Input: part model. Units: mm. Frame: model coordinates. A direction names the side the tool comes from. Give positions to 0.01 mm unless a question says otherwise; leave off trailing zeros. Write each loop counter-clockwise with the first axis right and the second up, starting at its lowest first coordinate (ties: lowest second). Pieces come first, ordered by that corner, then holes. Notation, with made-up numbers: (4.5, 44) - (39.5, 44) arc R19 cw to (39.5, 77) - close; hole circle Ø11 at (31, -15.5). An arc over 180 degrees is marked (long way). Use a Markdown table: item, result. Add a question column.
1. Section query D-D, the plane y = 29.5. Return loops of the section in (x, z).
2. Mould query, pull axis Y, two halves, no side actions, for faces 1 (the flat face through (-36, 20, 47)), 2 (the flat face through (-13, -22, 5)), 3 (the conical face through (-32.96, 35.88, 89.19)). Classes: released by +Y, released by -Y, zero draft, split by the parting line, or undercut.
3. Set-up query: faces 4 (the cylindrical face through (-7.262, -32.703, 45.56)), 5 (the cylindrical face through (2.769, -34.504, 9.677)), 6 (the flat face through (16, 30, 85)). Return all of +Z, -Z, +X, -X, +Y, -Y with unobstructed straight access to the full face (end or side cutting, diameter ignored); none if empty.
4. Pin query (flat end, axial travel): pin 1 (3 mm diameter, centred on x = 4, z = 16, fed in from -Y); pin 2 (2.5 mm diameter, centred on x = -31, z = 90, fed in from +Y); pin 3 (12 mm diameter, centred on x = 23, z = 40.5, fed in from -Y); pin 4 (5 mm diameter, centred on x = -3.5, z = 12.5, fed in from -Y). Return the tip coordinate at first contact, or that it passes through.
5. Section query A-A, the plane z = 90. Return loops of the section in (x, y), plus the area to 4 significant figures.
6. Material intervals for probe 1 along X at (y, z) = (37.1, 90); probe 2 along Y at (x, z) = (0, 30); probe 3 along Z at (x, y) = (-31, 37.4), sorted ascending.
7. Section query C-C, the plane y = 21. Return loops of the section in (x, z).
8. Section query B-B, the plane x = -31. Return loops of the section in (y, z), plus the area to 3 significant figures.
```python
from build123d import *
from build123d import SkipClean  # not in build123d's __all__

# Parameters (mm, degrees)
F1_DEPTH        = 95
F2_W            = 72
F2_H            = 80
F3_DEPTH        = 10
F4_R            = 33.5
F5_DEPTH        = 80
F7_D            = 4
F7_CSINK_D      = 9
F7_CSINK_ANGLE  = 90
F7_COPIES_COUNT = 2
F7_COPIES_PITCH = 81.154174
F8_R            = 25
F9_DEPTH        = 5.001
F11_R           = 6
F12_DEPTH       = 73.5


# Not quite as in the source:
# - a feature of the source that left no trace in its solid (it failed there, or was rolled back) is left out
# - a pattern or mirror of a feature is missing from the dataset's text; its kind, count and spacing are read off the source's solid


with BuildPart() as f1:
    # F0 (on Top) → F1 (new body)
    with BuildSketch(Plane.XY):
        with BuildLine():
            Line((36, 38.5), (-36, 38.5))
            Line((-36, 38.5), (-36, 0))
            ThreePointArc((-36, 0), (0, -36), (36, 0))
            Line((36, 0), (36, 38.5))
        make_face()
    extrude(amount=F1_DEPTH)

    # F2 (on face) → F3 (cut)
    with BuildSketch(Plane.XY.offset(95)):
        with Locations((0, -6.5)):
            Rectangle(F2_W, F2_H)
    extrude(amount=-F3_DEPTH, mode=Mode.SUBTRACT)

    # F4 (on face) → F5 (cut)
    with BuildSketch(Plane.XY.offset(85)):
        Circle(F4_R)
    extrude(amount=-F5_DEPTH, mode=Mode.SUBTRACT)

    # F7 (through all)
    with Locations(Plane.XZ.offset(-33.5)):
        with Locations((-31, 90), (31, 90)):
            f7 = CounterSinkHole(F7_D / 2, F7_CSINK_D / 2, counter_sink_angle=F7_CSINK_ANGLE)

    # F7_copies: F7 ×2
    with Locations(*[Vector(-0.3819889769, 0, -0.9241668797) * (i * F7_COPIES_PITCH) for i in range(1, F7_COPIES_COUNT)]):
        add(f7, clean=False, mode=Mode.SUBTRACT)

    # F8 (on face) → F9 (cut, through all)
    with BuildSketch(Plane.XY.offset(5)):
        Circle(F8_R)
    extrude(amount=-F9_DEPTH, mode=Mode.SUBTRACT)

    # F11 (on offset) → F12 (cut)
    with BuildSketch(Plane.XZ.offset(40)):
        with Locations((0, 15)):
            Circle(F11_R)
    with SkipClean():  # cleaning this boolean's faces spoils the solid; the shape is the same uncleaned
        extrude(amount=-F12_DEPTH, mode=Mode.SUBTRACT)


solid = f1.part
```
Result sheet:
| question | item | result |
|---|---|---|
| 1 | outline | (-36, 0) - (36, 0) - (36, 85) - (15.87, 85) - (15.87, 5) - (-15.87, 5) - (-15.87, 85) - (-36, 85) - close |
| 2 | face 1 | zero draft |
| 2 | face 2 | undercut |
| 2 | face 3 | released by -Y |
| 3 | face 4 | +Z |
| 3 | face 5 | -Y |
| 3 | face 6 | +Z, +X, -X, -Y |
| 4 | pin 1 | stops at y = 33.5 |
| 4 | pin 2 | passes through |
| 4 | pin 3 | stops at y = -31.73 |
| 4 | pin 4 | stops at y = -35.85 |
| 5 | outline | (-36, 33.5) - (-35.5, 33.5) - (-33, 36) - (-33, 38.5) - (-36, 38.5) - close; (-29, 36) - (-26.5, 33.5) - (26.5, 33.5) - (29, 36) - (29, 38.5) - (-29, 38.5) - close; (33, 36) - (35.5, 33.5) - (36, 33.5) - (36, 38.5) - (33, 38.5) - close |
| 5 | area | 307.5 mm² |
| 6 | probe 1 | x = -36 to -33, -29 to 29, 33 to 36 |
| 6 | probe 2 | y = -36 to -33.5, 33.5 to 38.5 |
| 6 | probe 3 | z = 0 to 88, 92 to 95 |
| 7 | outline | (-36, 0) - (-13.56, 0) - (-13.56, 5) - (-26.1, 5) - (-26.1, 85) - (-36, 85) - close; (13.56, 0) - (36, 0) - (36, 85) - (26.1, 85) - (26.1, 5) - (13.56, 5) - close |
| 8 | outline | (-18.3, 0) - (38.5, 0) - (38.5, 88) - (36, 88) - (33.5, 85.5) - (33.5, 85) - (12.7, 85) - (12.7, 5) - (-12.7, 5) - (-12.7, 85) - (-18.3, 85) - close; (33.5, 94.5) - (36, 92) - (38.5, 92) - (38.5, 95) - (33.5, 95) - close |
| 8 | area | 2,820 mm² |
